The drawing under review shows one solid part. Ordinate dimensions are in mm from its lowest x, y, z. A direction names the side the tool comes from. Give positions to 0.01 mm unless a question says otherwise; leave off trailing zeros. Write each loop counter-clockwise with the first axis right and the second up, starting at its lowest first coordinate (ties: lowest second). Pieces come first, ordered by that corner, then holes.
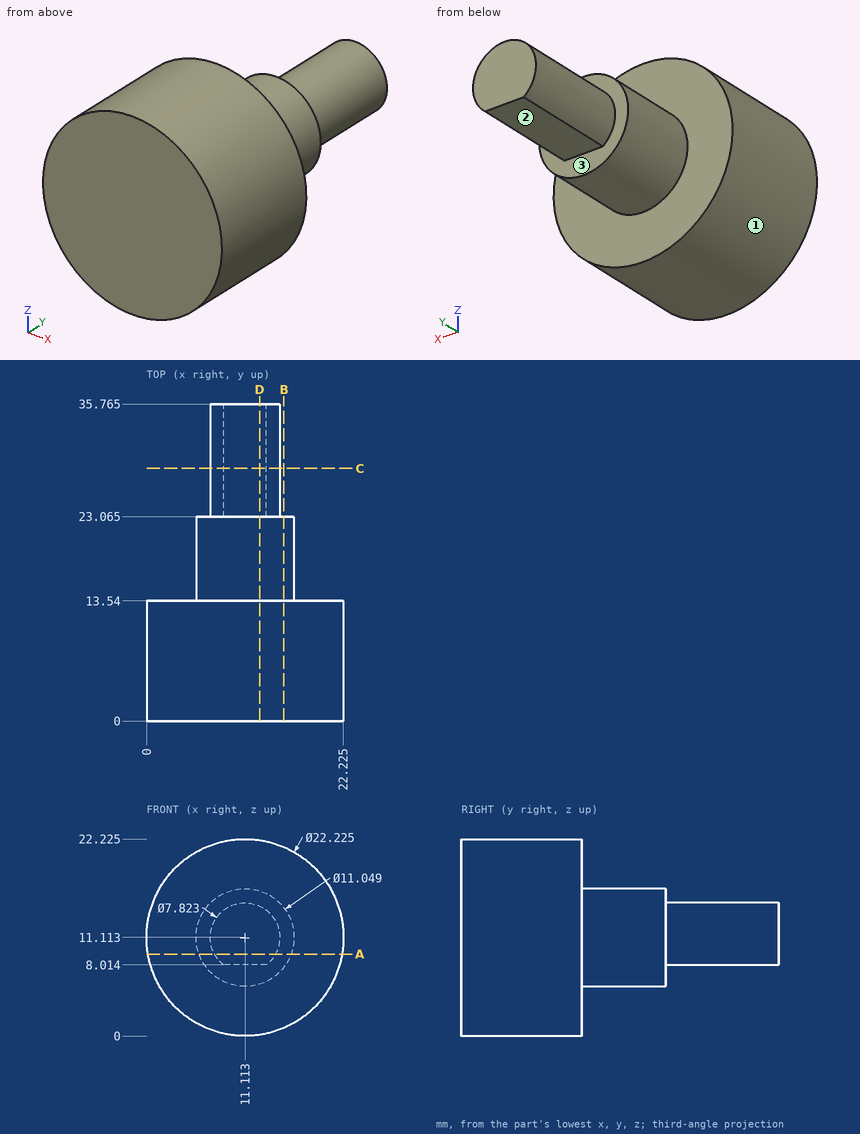
1) To check wall thickness, follow probe 1 along Y at (x, z) = (11.75, 17); probe 2 along Y at (x, z) = (9.75, 16.25) (1 decimal); probe 3 along X at (y, z) = (17, 11) (1 decimal). State the ranges of each line that lie inside material, in increasing order.
2) Insertion check: pin 1 (1.4 mm diameter, centred on x = 11.5, y = 31, fed in from -Z); pin 2 (12 mm diameter, centred on y = 28, z = 10.5, fed in from -X); pin 3 (5 mm diameter, centred on x = 9.5, z = 3, fed in from +Y). Each pin has a flat end and moves straight along its axis. Give the tip position at first contact, or say it passes through.
3) Tool access review of the marked faces 1, 2 and 3: name each direction out of +Z, -Z, +X, -X, +Y, -Y from which nothing blocks a thin tool from reaching the whole face with its end or side.
4) Consider section D-D, the plane x = 12.75. Give the boundary of the cut face in (y, z) (1 decimal).
5) Consider section C-C, the plane y = 28.5. Give the boundary of the cut face in (x, z) (1 decimal), then the cut area to 3 significant figures.
6) Consider section B-B, the plane x = 15.5. Give the boundary of the cut face in (y, z) (1 decimal).
7) Consider section A-A, the plane z = 9.25. Give the boundary of the cut face in (x, y) (1 decimal).
Answer block:
1. probe 1: y = 0 to 13.54
1. probe 2: y = 0 to 23.1
1. probe 3: x = 5.6 to 16.6
2. pin 1: stops at z = 8.01
2. pin 2: stops at x = 5.59
2. pin 3: stops at y = 13.54
3. face 1: +Y, -Y
3. face 2: -Z, +X, -X, +Y
3. face 3: +Y
4. outline: (0, 0.1) - (13.5, 0.1) - (13.5, 5.8) - (23.1, 5.8) - (23.1, 8) - (35.8, 8) - (35.8, 14.7) - (23.1, 14.7) - (23.1, 16.4) - (13.5, 16.4) - (13.5, 22.1) - (0, 22.1) - close
5. outline: (8.7, 8) - (13.5, 8) arc R3.9 ccw (long way) to start
5. area: 45.4 mm2
6. outline: (0, 0.9) - (13.5, 0.9) - (13.5, 7.8) - (23.1, 7.8) - (23.1, 14.5) - (13.5, 14.5) - (13.5, 21.3) - (0, 21.3) - close
7. outline: (0.2, 0) - (22.1, 0) - (22.1, 13.5) - (16.3, 13.5) - (16.3, 23.1) - (14.6, 23.1) - (14.6, 35.8) - (7.7, 35.8) - (7.7, 23.1) - (5.9, 23.1) - (5.9, 13.5) - (0.2, 13.5) - close
